Verification items for the finished model (mm, model axes). A direction names the side the tool comes from. Coordinates: 2 decimals unless noted, no trailing zeros. Order: outer loops, then holes, each group sorted by start corner. A loop starts at its lowest first (then second) coordinate and runs counter-clockwise, first axis right, second up. Notation, with made-up numbers: (22.5, -16.75) -> (47.5, -16.75) arc R6 cw to (47.5, -9.75) -> close; hole circle Ø5 at (-35, 81.25). An arc over 180 degrees is marked (long way). Write item = value, one per line. Start each with the question number.
1. Cross-section at A-A on y = 16.5. Record the cut outline in (x, z) (3 decimals).
2. Cross-section at C-C on z = 0. Record the cut outline in (x, y) (3 decimals).
3. Cross-section at D-D on z = 9. Record the cut outline in (x, y) (3 decimals), plus the area to 3 significant figures.
4. Go/stop test with flat-tipped pins: P1, Ø15, axis at x = 20.5, z = -25, coming from the +Y side; P2, Ø6, axis at x = -23.57, z = 23.57, coming from the -Y side; P3, Ø2, axis at y = -1.5, z = 4, coming from the -X side; P4, Ø2, axis at x = 25, y = 26.5, coming from the +Z side. Record where each tip stops, or that it passes through.
5. Release check for a two-part mould opening along X. For faces 5 (the flat face through (7, 0.5, -18)), 6 (the cylindrical face through (17.12, 40.2, 27.72)), 7 (the flat face through (0, 76.2, 0)) record: +X half, -X half, draft (parallel to the pull), parting line (faces both ways), or undercut.
6. Thickness scan on line 1 along Z through (x, y) = (-23.57, 2.15) (3 decimals); line 2 along Z through (x, y) = (-23, 1) (3 decimals); line 3 along Y through (x, z) = (-14, -8). Record the ranges inside material, lowest first. Write a range as from..to.
7. Set-up check for faces 1 (the cylindrical face through (-0.69, -9.85, -3.1)), 2 (the cylindrical face through (19.69, 41.2, 19.6)), 3 (the flat face through (-25, 41, -18.02)), 4 (the flat face through (-25, 41, 18.02)): record each of +Z, -Z, +X, -X, +Y, -Y from which the full face is reachable in a straight line by a thin tool's end or side.
8. Cross-section at B-B on x = 0. Record the cut outline in (y, z) (3 decimals).
from build123d import *

# Parameters (mm, degrees)
F0_W      = 57.15
F0_H      = 57.15
F1_DEPTH  = 76.2
F2_R      = 2.5
F3_DEPTH  = 76.201
F5_DEPTH  = 71
F6_R      = 3
F7_R      = 24.125
F8_DEPTH  = 0.5
F9_R      = 19
F9_R_2    = 13.5
F10_DEPTH = 2
F11_R     = 3.175
F12_DEPTH = 21


with BuildPart() as f1:
    # F0 (on Front) → F1 (new body)
    with BuildSketch(Plane.XZ):
        Rectangle(F0_W, F0_H)
    extrude(amount=-F1_DEPTH)

    # F2 (on face) → F3 (cut, through all)
    with BuildSketch(Plane.XZ):
        with Locations((-23.57, 23.57)):
            Circle(F2_R)
        with Locations((23.57, 23.57)):
            Circle(F2_R)
        with Locations((-23.57, -23.57)):
            Circle(F2_R)
        with Locations((23.57, -23.57)):
            Circle(F2_R)
    extrude(amount=-F3_DEPTH, mode=Mode.SUBTRACT)

    # F4 (on face) → F5 (cut)
    with BuildSketch(Plane(origin=(0, 76.2, 0), x_dir=(-1, 0, 0), z_dir=(0, 1, 0))):
        with BuildLine():
            Line((-28.575, 18.02), (-23.57, 18.02))
            ThreePointArc((-23.57, 18.02), (-19.6455573644, 19.6455573644), (-18.02, 23.57))
            Line((-18.02, 23.57), (-18.02, 28.575))
            Line((-18.02, 28.575), (-28.575, 28.575))
            Line((-28.575, 28.575), (-28.575, 18.02))
        make_face()
        with BuildLine():
            Line((18.02, 28.575), (18.02, 23.57))
            ThreePointArc((18.02, 23.57), (19.6455573644, 19.6455573644), (23.57, 18.02))
            Line((23.57, 18.02), (28.575, 18.02))
            Line((28.575, 18.02), (28.575, 28.575))
            Line((28.575, 28.575), (18.02, 28.575))
        make_face()
        with BuildLine():
            ThreePointArc((23.57, -18.02), (19.6455573644, -19.6455573644), (18.02, -23.57))
            Line((18.02, -23.57), (18.02, -28.575))
            Line((18.02, -28.575), (28.575, -28.575))
            Line((28.575, -28.575), (28.575, -18.02))
            Line((28.575, -18.02), (23.57, -18.02))
        make_face()
        with BuildLine():
            ThreePointArc((-18.02, -23.57), (-19.6455573644, -19.6455573644), (-23.57, -18.02))
            Line((-23.57, -18.02), (-28.575, -18.02))
            Line((-28.575, -18.02), (-28.575, -28.575))
            Line((-28.575, -28.575), (-18.02, -28.575))
            Line((-18.02, -28.575), (-18.02, -23.57))
        make_face()
    extrude(amount=-F5_DEPTH, mode=Mode.SUBTRACT)

    # F6
    f6_edges = [f1.edges().sort_by_distance(p)[0] for p in [
        (-18.02, 40.7, 28.575),
        (-28.575, 40.7, 18.02),
        (-28.575, 2.6, 28.575),
        (28.575, 2.6, 28.575),
        (18.02, 40.7, 28.575),
        (28.575, 40.7, 18.02),
        (-28.575, 2.6, -28.575),
        (-28.575, 40.7, -18.02),
        (-18.02, 40.7, -28.575),
        (28.575, 2.6, -28.575),
        (28.575, 40.7, -18.02),
        (18.02, 40.7, -28.575),
    ]]
    fillet(f6_edges, radius=F6_R)

    # F7 (on face) → F8 (cut)
    with BuildSketch(Plane.XZ):
        Circle(F7_R)
    extrude(amount=-F8_DEPTH, mode=Mode.SUBTRACT)

    # F9 (on face) → F10 (join)
    with BuildSketch(Plane.XZ.offset(-0.5)):
        Circle(F9_R)
        Circle(F9_R_2, mode=Mode.SUBTRACT)
    extrude(amount=F10_DEPTH)

    # F11 (on face) → F12 (join)
    with BuildSketch(Plane.XZ.offset(-0.5)):
        Circle(F11_R)
    extrude(amount=F12_DEPTH)


solid = f1.part
Worked out:
q1.outline = (-28.575, -15.02) arc R3 ccw to (-25.575, -18.02) -> (-23.57, -18.02) arc R5.55 cw to (-18.02, -23.57) -> (-18.02, -25.575) arc R3 ccw to (-15.02, -28.575) -> (15.02, -28.575) arc R3 ccw to (18.02, -25.575) -> (18.02, -23.57) arc R5.55 cw to (23.57, -18.02) -> (25.575, -18.02) arc R3 ccw to (28.575, -15.02) -> (28.575, 15.02) arc R3 ccw to (25.575, 18.02) -> (23.57, 18.02) arc R5.55 cw to (18.02, 23.57) -> (18.02, 25.575) arc R3 ccw to (15.02, 28.575) -> (-15.02, 28.575) arc R3 ccw to (-18.02, 25.575) -> (-18.02, 23.57) arc R5.55 cw to (-23.57, 18.02) -> (-25.575, 18.02) arc R3 ccw to (-28.575, 15.02) -> close
q2.outline = (-28.575, 0) -> (-24.125, 0) -> (-24.125, 0.5) -> (-19, 0.5) -> (-19, -1.5) -> (-13.5, -1.5) -> (-13.5, 0.5) -> (-3.175, 0.5) -> (-3.175, -20.5) -> (3.175, -20.5) -> (3.175, 0.5) -> (13.5, 0.5) -> (13.5, -1.5) -> (19, -1.5) -> (19, 0.5) -> (24.125, 0.5) -> (24.125, 0) -> (28.575, 0) -> (28.575, 76.2) -> (-28.575, 76.2) -> close
q3.outline = (-28.575, 0) -> (-22.383, 0) -> (-22.383, 0.5) -> (-16.733, 0.5) -> (-16.733, -1.5) -> (-10.062, -1.5) -> (-10.062, 0.5) -> (10.062, 0.5) -> (10.062, -1.5) -> (16.733, -1.5) -> (16.733, 0.5) -> (22.383, 0.5) -> (22.383, 0) -> (28.575, 0) -> (28.575, 76.2) -> (-28.575, 76.2) -> close
q3.area = 4,360 mm²
q4.P1 = 76.2
q4.P2 = 0
q4.P3 = -18.76
q4.P4 = 18.02
q5.face_5 = undercut
q5.face_6 = +X half
q5.face_7 = draft
q6.line_1 = -28.575..-26.07, -21.07..21.07, 26.07..28.575
q6.line_2 = -28.575..-26.004, -21.136..21.136, 26.004..28.575
q6.line_3 = -1.5..76.2
q7.face_1 = -Y
q7.face_2 = +Z, +X, +Y
q7.face_3 = -Z, -X, +Y
q7.face_4 = +Z, -X, +Y
q8.outline = (-20.5, -3.175) -> (0.5, -3.175) -> (0.5, -13.5) -> (-1.5, -13.5) -> (-1.5, -19) -> (0.5, -19) -> (0.5, -24.125) -> (0, -24.125) -> (0, -28.575) -> (76.2, -28.575) -> (76.2, 28.575) -> (0, 28.575) -> (0, 24.125) -> (0.5, 24.125) -> (0.5, 19) -> (-1.5, 19) -> (-1.5, 13.5) -> (0.5, 13.5) -> (0.5, 3.175) -> (-20.5, 3.175) -> close
